Build history of the part. All positions in model axes, mm. Give positions to 0.01 mm unless a question says otherwise; leave off trailing zeros. Order: outer loops, then holes, each group sorted by start corner. A loop starts at its lowest first (then second) coordinate and runs counter-clockwise, first axis right, second up. Notation, with made-up numbers: M -3.5,48.25 L 42.5,48.25 A24 ccw 42.5,85.25 Z; hole C -7,-0.5 d10. An arc over 180 degrees is marked long. One line per item, written item: value.
Autodesk Inventor part; units mm, degrees
ref_plane "YZ Plane" through (0, 0, 0) normal (1, 0, 0) x (0, 1, 0)
ref_plane "XZ Plane" through (0, 0, 0) normal (0, 1, 0) x (-1, 0, 0)
ref_plane "XY Plane" through (0, 0, 0) normal (0, 0, 1) x (1, 0, 0)
sketch "Sketch8" plane through (0, 0, 0) normal (0, 0, 1) x (1, 0, 0)
  arc A0 (0, -38.1) -> (0, 38.1) centre (0, 0) ccw
  line L0 (0, 38.1) -> (0, -38.1)
  line L1 (0, -53.34) -> (0, 53.34)
  dimension "d25" = 76.2
revolve "Revolution1" add sketch "Sketch8" angle 360 about axis through (0, -10, 0) along (0, 1, 0)
sketch "Sketch9" plane through (0, 0, 0) normal (0, 1, 0) x (-1, 0, 0)
  circle A0 centre (0, 0) radius 6.35
  dimension "d27" = 12.7
extrude "Extrusion4" cut sketch "Sketch9" along normal mid plane 76.2
fillet "Fillet1" radius 3.175 4 edges at (0, 37.5671, 6.35) (0, 37.5671, -6.35) (0, -37.5671, -6.35) (0, -37.5671, 6.35)
equation "\"d25\" = ballDiam"
equation "\"d27\" = holeDiam"
equation "\"d28\" = ballDiam"
equation "\"ballDiam\" = 76.2"
equation "\"holeDiam\" = 12.7"
properties part number "float"
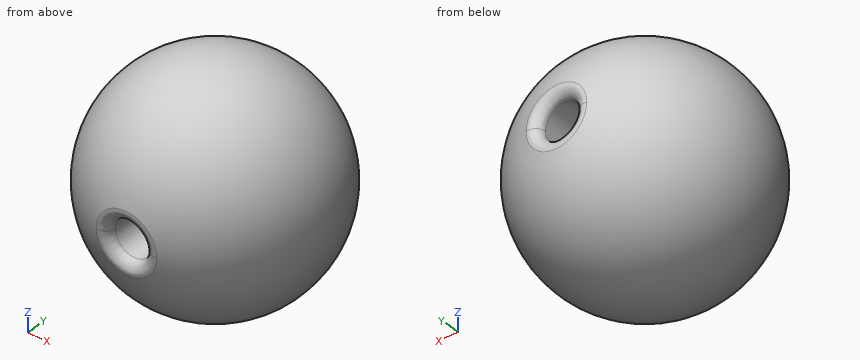
1) Saw through at C-C, the plane z = 32.5. Write the cut outline in (x, y), then the cut area to 3 significant figures.
Check values:
outline: C 0,0 d39.77
area: 1,240 mm^2
2) Saw through at D-D, the plane y = 22.5. Write the cut outline in (x, z).
Check values:
outline: C 0,0 d61.49; hole C 0,0 d12.7
3) Drill centre lines: probe 1 along X at (y, z) = (0, 0); probe 2 along Z at (x, y) = (0, 5.5); probe 3 along Z at (x, y) = (0, 2). Where is each one in solid material? Low to high. Write a range as from..to.
Check values:
probe 1: -38.1..-6.35, 6.35..38.1
probe 2: -37.7..-6.35, 6.35..37.7
probe 3: -38.05..-6.35, 6.35..38.05
4) Pin check, flat tips, straight feed: pin 1 (3 mm diameter, centred on x = 11, y = -15.5, fed in from -Z); pin 2 (1 mm diameter, centred on x = -22.5, z = -11, fed in from -Y); pin 3 (12 mm diameter, centred on x = 11.5, y = 25, fed in from -Z). Stop position of each tip, or through.
Check values:
pin 1: z = -33.84
pin 2: y = -29.14
pin 3: z = -31.44
5) Saw through at B-B, the plane x = -15.5. Write the cut outline in (y, z).
Check values:
outline: C 0,0 d69.61
6) Saw through at A-A, the plane y = 12.5. Write the cut outline in (x, z), then the cut area to 3 significant figures.
Check values:
outline: C 0,0 d71.98; hole C 0,0 d12.7
area: 3,940 mm^2
